Read the model definition and answer for the solid it produces. Units are mm, in the model's axes. Coordinates: 2 decimals unless noted, no trailing zeros. Write each loop counter-clockwise with the first axis right and the second up, starting at its lowest first coordinate (ties: lowest second). Pieces come first, ordered by that corner, then holes.
1) Each of these flat-tipped pins is pushed along its axis until it touches: pin 1 Ø1.2 at (x, z) = (5, 1.5) entering from -Y; pin 2 Ø0.5 at (x, z) = (6, 6) entering from +Y. Where does it stop, or does it pass through?
2) Find the intervals of material crossed by line 1 (Y direction, x = 5.25, z = 1.75), in increasing order.
3) The part is cut by section A-A (z = 1). Determine the outline of the cut face in (x, y), then the cut area to 3 significant figures.
from build123d import *

# Parameters (mm, degrees)
BOSS_EXTRUDE1_DEPTH = 6.2
CUT_EXTRUDE1_DEPTH  = 1


with BuildPart() as part:
    # Sketch2 → Boss-Extrude1 (new body)
    with BuildSketch(Plane.XY):
        Polygon((0, 0), (0, 186.19), (3, 186.19), (3, 179.99), (7, 179.99), (7, 186.19), (10, 186.19), (10, 0), (7, 0), (7, 6.2), (3, 6.2), (3, 0), align=None)
    extrude(amount=BOSS_EXTRUDE1_DEPTH)

    # Sketch3 → Cut-Extrude1 (cut)
    with BuildSketch(Plane.XY.offset(6.2)):
        with BuildLine():
            Line((3.072648213, 30.209362795), (2.844953902, 30.367731185))
            Line((2.844953902, 30.367731185), (3.72774637, 31.658210953))
            add(Edge.make_bspline(
                [(3.72774637, 31.658210953), (3.671421203, 31.651322959), (3.560513808, 31.637760117), (3.448810866, 31.635268509), (3.393837115, 31.634042283)],
                knots=[0, 0, 0, 0, 0.000170115, 0.000334967, 0.000334967, 0.000334967, 0.000334967], degree=3))
            add(Edge.make_bspline(
                [(3.393837115, 31.634042283), (3.360506829, 31.634895973), (3.295082392, 31.636571694), (3.198896536, 31.649853906), (3.106471777, 31.670310093), (3.018053147, 31.700834321), (2.933308311, 31.73876941), (2.852422271, 31.78581113), (2.775503913, 31.841152552), (2.703379334, 31.904501051), (2.637782256, 31.974058999), (2.579341122, 32.04767876), (2.530771667, 32.126215534), (2.49042505, 32.208067233), (2.45982671, 32.294410316), (2.437544979, 32.384262271), (2.423826844, 32.478252832), (2.422194807, 32.542229201), (2.421366162, 32.574712355)],
                knots=[0, 0, 0, 0, 9.9954e-05, 0.000196201, 0.000290782, 0.000383503, 0.000476303, 0.000568919, 0.000663705, 0.000760153, 0.000856434, 0.000950205, 0.001041624, 0.001132931, 0.001223461, 0.001315861, 0.001410305, 0.001507717, 0.001507717, 0.001507717, 0.001507717], degree=3))
            add(Edge.make_bspline(
                [(2.421366162, 32.574712355), (2.422939542, 32.619133918), (2.426027768, 32.706324436), (2.450882137, 32.833717927), (2.491758302, 32.954174291), (2.548752615, 33.067376824), (2.620539113, 33.171697109), (2.706816191, 33.265684919), (2.807059073, 33.348003465), (2.91898419, 33.418764307), (3.03995443, 33.475673911), (3.166653856, 33.517619562), (3.298111665, 33.542292712), (3.387163766, 33.5455456), (3.431998173, 33.547183308)],
                knots=[0, 0, 0, 0, 0.000133185, 0.000261414, 0.000387724, 0.00051373, 0.000640399, 0.00076644, 0.000895188, 0.001028407, 0.001162697, 0.001295241, 0.001427846, 0.0015623, 0.0015623, 0.0015623, 0.0015623], degree=3))
            add(Edge.make_bspline(
                [(3.431998173, 33.547183308), (3.475984097, 33.545523089), (3.562896136, 33.542242652), (3.690702591, 33.518217909), (3.813113371, 33.47772607), (3.929449895, 33.421769358), (4.037163504, 33.351628249), (4.134024419, 33.268049074), (4.217822229, 33.170979774), (4.288419607, 33.062768073), (4.345088858, 32.946502311), (4.385975857, 32.825141182), (4.411145116, 32.699557484), (4.414316784, 32.614472497), (4.415917444, 32.571532267)],
                knots=[0, 0, 0, 0, 0.000131915, 0.000260652, 0.000388569, 0.000517718, 0.000646848, 0.000773094, 0.000900237, 0.001030248, 0.001159674, 0.001287189, 0.001413545, 0.001542287, 0.001542287, 0.001542287, 0.001542287], degree=3))
            add(Edge.make_bspline(
                [(4.415917444, 32.571532267), (4.414848459, 32.538200421), (4.41268029, 32.470595109), (4.397498068, 32.367879012), (4.3717169, 32.263148254), (4.342460002, 32.174500806), (4.314218678, 32.101286713), (4.287638366, 32.043454922), (4.258145198, 31.982584491), (4.223747461, 31.919313691), (4.186770235, 31.852835963), (4.144987891, 31.783818071), (4.099353551, 31.712167398), (4.066850877, 31.663864683), (4.050207308, 31.639130424)],
                knots=[0, 0, 0, 0, 9.9984e-05, 0.000202793, 0.000310776, 0.000423207, 0.000482616, 0.000546097, 0.000614079, 0.0006855, 0.000762103, 0.000842274, 0.000927493, 0.001016928, 0.001016928, 0.001016928, 0.001016928], degree=3))
            Line((4.050207308, 31.639130424), (3.072648213, 30.209362795))
        make_face()
        with BuildLine():
            add(Edge.make_bspline(
                [(3.446626579, 31.959683308), (3.471876006, 31.960373085), (3.521028056, 31.961715846), (3.593034606, 31.969888515), (3.661001562, 31.984379203), (3.725110481, 32.005170656), (3.786004171, 32.030259205), (3.842715411, 32.062201507), (3.895291665, 32.100316597), (3.944084999, 32.143142826), (3.98741377, 32.190722998), (4.026006377, 32.240522516), (4.058809177, 32.292759984), (4.08472015, 32.348089586), (4.106024015, 32.405164482), (4.120736069, 32.46490379), (4.128886142, 32.526996268), (4.1302755, 32.569177193), (4.130981547, 32.590612795)],
                knots=[0, 0, 0, 0, 7.5753e-05, 0.000147465, 0.000217073, 0.000283852, 0.000349411, 0.000414338, 0.000478589, 0.000543925, 0.000608743, 0.000671332, 0.000732749, 0.000793345, 0.000854313, 0.000915245, 0.00097749, 0.001041807, 0.001041807, 0.001041807, 0.001041807], degree=3))
            add(Edge.make_bspline(
                [(4.130981547, 32.590612795), (4.130374061, 32.612057349), (4.129176936, 32.654316472), (4.119572743, 32.716500879), (4.102677005, 32.776094051), (4.080007065, 32.833422241), (4.050143706, 32.888014436), (4.014308401, 32.940556034), (3.971733965, 32.990713892), (3.922745923, 33.037308363), (3.869918864, 33.080259672), (3.813621124, 33.118165612), (3.754316736, 33.14993484), (3.692367506, 33.176150334), (3.627644361, 33.196608017), (3.5601856, 33.211319483), (3.48965034, 33.219458146), (3.441770173, 33.220838722), (3.417369768, 33.221542283)],
                knots=[0, 0, 0, 0, 6.4316e-05, 0.000126743, 0.000188161, 0.000249812, 0.000311283, 0.000374438, 0.00044032, 0.000508243, 0.00057698, 0.000644365, 0.000711521, 0.0007785, 0.000845884, 0.000914871, 0.00098532, 0.001058531, 0.001058531, 0.001058531, 0.001058531], degree=3))
            add(Edge.make_bspline(
                [(3.417369768, 33.221542283), (3.393181571, 33.220837585), (3.34572453, 33.219454975), (3.275816328, 33.211334953), (3.208813697, 33.196509078), (3.144278084, 33.17615981), (3.082330695, 33.149932885), (3.023029104, 33.118163947), (2.966718196, 33.080268397), (2.913941785, 33.037274568), (2.864867241, 32.990930775), (2.823024797, 32.940336307), (2.787107481, 32.888041767), (2.757285157, 32.833414977), (2.734604302, 32.77609599), (2.717711486, 32.716500354), (2.708106508, 32.654316609), (2.70690949, 32.612057395), (2.706302059, 32.590612795)],
                knots=[0, 0, 0, 0, 7.2576e-05, 0.000142393, 0.000210758, 0.000278143, 0.000345121, 0.000412278, 0.000479663, 0.0005484, 0.000616323, 0.000681795, 0.00074495, 0.000806421, 0.000868072, 0.00092949, 0.000991917, 0.001056233, 0.001056233, 0.001056233, 0.001056233], degree=3))
            add(Edge.make_bspline(
                [(2.706302059, 32.590612795), (2.706851721, 32.569160501), (2.707935754, 32.52685265), (2.718393106, 32.464689422), (2.73588126, 32.405100846), (2.759303136, 32.347507519), (2.790147435, 32.292469476), (2.827996926, 32.240247655), (2.872361243, 32.190250068), (2.922647335, 32.143253526), (2.977682024, 32.100116909), (3.036461929, 32.06244292), (3.097975139, 32.030627203), (3.162438189, 32.005098947), (3.229373358, 31.984586938), (3.299382227, 31.969915222), (3.372233271, 31.961794237), (3.421590897, 31.960393702), (3.446626579, 31.959683308)],
                knots=[0, 0, 0, 0, 6.4316e-05, 0.000126844, 0.000188436, 0.000250326, 0.000312966, 0.000377217, 0.000443451, 0.000513196, 0.000583426, 0.000652939, 0.000722346, 0.000790847, 0.000860662, 0.000932137, 0.001005113, 0.00108023, 0.00108023, 0.00108023, 0.00108023], degree=3))
        make_face(mode=Mode.SUBTRACT)
        Polygon((5.026494367, 33.465773052), (6.980340521, 33.465773052), (5.311430264, 30.209362795), (5.065291442, 30.34483455), (6.498239159, 33.140132026), (5.026494367, 33.140132026), align=None)
    extrude(amount=-CUT_EXTRUDE1_DEPTH, mode=Mode.SUBTRACT)


solid = part.part
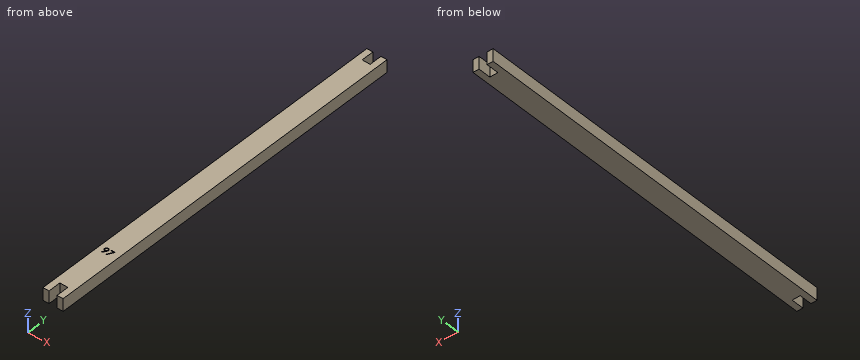
Reported:
1. pin 1: stops at y = 6.2
1. pin 2: stops at y = 179.99
2. line 1: y = 6.2 to 179.99
3. outline: (0, 0) - (3, 0) - (3, 6.2) - (7, 6.2) - (7, 0) - (10, 0) - (10, 186.19) - (7, 186.19) - (7, 179.99) - (3, 179.99) - (3, 186.19) - (0, 186.19) - close
3. area: 1,810 mm2
